from build123d import *

# Parameters (mm, degrees)
F0_R     = 3
F1_DEPTH = 3
F2_SIZE  = 1
F3_DEPTH = 25
F4_DEPTH = 10
F5_SIZE  = 1


with BuildPart() as f1:
    # F0 (on Front) → F1 (new body)
    with BuildSketch(Plane.XZ):
        with BuildLine():
            ThreePointArc((2.3094010768, 4), (0, 4.6188021535), (-2.3094010768, 4))
            Line((-2.3094010768, 4), (2.3094010768, 4))
        make_face()
        Polygon((2.3094010768, 4), (-2.3094010768, 4), (-4.6188021535, 0), (-2.3094010768, -4), (2.3094010768, -4), (4.6188021535, 0), align=None)
        Circle(F0_R, mode=Mode.SUBTRACT)
        with BuildLine():
            Line((-4.6188021535, 0), (-2.3094010768, 4))
            ThreePointArc((-2.3094010768, 4), (-4, 2.3094010768), (-4.6188021535, 0))
        make_face()
        with BuildLine():
            ThreePointArc((4.6188021535, 0), (4, 2.3094010768), (2.3094010768, 4))
            Line((2.3094010768, 4), (4.6188021535, 0))
        make_face()
        with BuildLine():
            Line((-2.3094010768, -4), (-4.6188021535, 0))
            ThreePointArc((-4.6188021535, 0), (-4, -2.3094010768), (-2.3094010768, -4))
        make_face()
        with BuildLine():
            ThreePointArc((2.3094010768, -4), (4, -2.3094010768), (4.6188021535, 0))
            Line((4.6188021535, 0), (2.3094010768, -4))
        make_face()
        with BuildLine():
            Line((2.3094010768, -4), (-2.3094010768, -4))
            ThreePointArc((-2.3094010768, -4), (0, -4.6188021535), (2.3094010768, -4))
        make_face()
        Circle(F0_R)
    extrude(amount=F1_DEPTH)

    # F2
    f2_edges = [f1.edges().sort_by_distance(p)[0] for p in [
        (2.309401, -3, 4),
    ]]
    chamfer(f2_edges, length=F2_SIZE)

    # F0 (on Front) → F3 (intersect)
    with BuildSketch(Plane.XZ):
        Polygon((2.3094010768, 4), (-2.3094010768, 4), (-4.6188021535, 0), (-2.3094010768, -4), (2.3094010768, -4), (4.6188021535, 0), align=None)
        Circle(F0_R, mode=Mode.SUBTRACT)
        Circle(F0_R)
    extrude(amount=F3_DEPTH, mode=Mode.INTERSECT)

    # F0 (on Front) → F4 (join)
    with BuildSketch(Plane.XZ):
        Circle(F0_R)
    extrude(amount=-F4_DEPTH)

    # F5
    f5_edges = [f1.edges().sort_by_distance(p)[0] for p in [
        (-3, 10, 0),
    ]]
    chamfer(f5_edges, length=F5_SIZE)


solid = f1.part
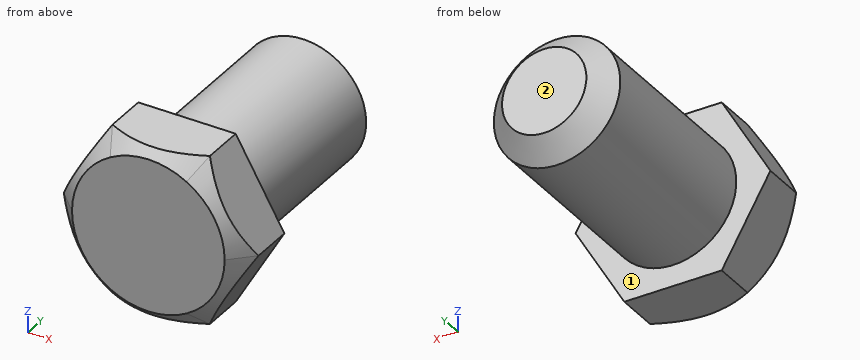
Model file for the job. Use its own axes, mm. Face numbers are marked on the shaded views. A direction names the side the tool comes from. Give positions to 0.01 mm unless a question says otherwise; leave off trailing zeros. Write each loop counter-clockwise with the first axis right and the second up, starting at its lowest first coordinate (ties: lowest second). Pieces come first, ordered by that corner, then holes. Notation, with made-up numbers: M 76,88.25 L 94,88.25 A28 ccw 94,111.25 Z; hole C 66.25,-30 d11. An arc over 180 degrees is marked long. One line per item, written item: value. Start each with the question number.
Q1. Drop flat-ended pins along their axis: pin 1 Ø3 at (x, y) = (-1.5, 7.5) entering from +Z; pin 2 Ø3 at (y, z) = (6, -2.5) entering from +X; pin 3 Ø1 at (y, z) = (-0.5, 2.5) entering from -X. Give the stop position or say it passes through.
Q2. Probe probe 1 along Z at (x, y) = (0, 7); probe 2 along Z at (x, y) = (1.5, 9.5); probe 3 along Y at (x, z) = (3, -2). List the from-to ranges inside material, lowest first. Write a range as [from, to].
Q3. 3-axis set-ups, long thin cutter, end or side, ignore diameter. For the marked faces 1 and 2: which of +Z, -Z, +X, -X, +Y, -Y reach the whole face in a straight line?
Q4. Saw through at A-A, the plane x = 0. Write the cut outline in (y, z).
Q5. Saw through at B-B, the plane y = 5. Write the cut outline in (x, z).
Output values:
1. pin 1: stops at z = 3
1. pin 2: stops at x = 2.83
1. pin 3: stops at x = -3.46
2. probe 1: z = [-3, 3]
2. probe 2: z = [-2, 2]
2. probe 3: y = [-3, 0]
3. face 1: +Y
3. face 2: +Z, -Z, +X, -X, +Y
4. outline: M -3,-3.62 L -2.62,-4 L 0,-4 L 0,-3 L 9,-3 L 10,-2 L 10,2 L 9,3 L 0,3 L 0,4 L -2.62,4 L -3,3.62 Z
5. outline: C 0,0 d6
